Read the model definition and answer for the solid it produces. Units are mm, in the model's axes. A direction names the side the tool comes from. Coordinates: 2 decimals unless noted, no trailing zeros. Write each loop counter-clockwise with the first axis right and the second up, starting at its lowest first coordinate (ties: lowest second). Pieces come first, ordered by that corner, then holes. Notation, with made-up numbers: (-9, -15) -> (13, -15) arc R11 ccw to (13, 3) -> close; hole circle Ø6 at (-37.75, 82). An arc over 180 degrees is marked (long way). Write item = value, one per line. Start each with the question number.
1) For a pull along Y with two mould halves and no side action, classify faces 1 (the face through (0, 0, 0)), 2 (the face through (5, 14.5, -2)) as released by +Y, released by -Y, zero draft, split by the parting line, or undercut.
2) Find the intervals of material crossed by line 1 along Y through (x, z) = (-7, -5.25); line 2 along Z through (x, y) = (6.25, 7.75); line 3 along X through (y, z) = (5.25, 0.5), in increasing order. Write a range as from..to.
3) Section B-B (y = 20.25) is taken. Determine the outline of the cut face in (x, z).
4) Section A-A (y = 11.5) is taken. Determine the outline of the cut face in (x, z), plus the area to 3 significant figures.
5) Flat-ended cylindrical pins translate along their axes: pin 1 Ø3 at (y, z) = (4.5, -1) entering from +X; pin 2 Ø1.5 at (x, y) = (1, 14) entering from +Z; pin 3 Ø8 at (y, z) = (7, -7) entering from -X. Find the tip coordinate at first contact, or state that the pin passes through.
6) A tool of negligible diameter and unlimited length cuts with its end or side. For faces 3 (the face through (7.606, 21.05, 9.92)), 4 (the face through (-6.324, 16.965, -4.032)), 5 (the face through (3.83, 1.275, -9.237)), from which of +Z, -Z, +X, -X, +Y, -Y can it reach the whole face along a straight path? Write none if from no direction.
from build123d import *

# Parameters (mm, degrees)
DOME1_FACE_RADIUS = 12.5
DOME1_HEIGHT      = 1
FILLET1_R         = 1


with BuildPart() as part:
    # Sketch1 → Revolve1 (revolve)
    with BuildSketch(Plane.XY, mode=Mode.PRIVATE) as revolve1_sk:
        Polygon((0, 23.5), (12.5, 23.5), (12.5, 19.5), (7.5, 19.5), (7.5, 14.5), (5, 14.5), (5, 10), (8, 10), (8, 5), (10, 3), (10, 0), (0, 0), align=None)
    revolve(revolve1_sk.sketch.rotate(Axis((0, 0, 0), (0, 1, 0)), 90), axis=Axis((0, 0, 0), (0, 1, 0)))

    # Dome1: a dome of height H over a round flat face of radius A is a cap of a sphere of radius (A * A + H * H) / (2 * H)
    dome1_r = (DOME1_FACE_RADIUS * DOME1_FACE_RADIUS + DOME1_HEIGHT * DOME1_HEIGHT) / (2 * DOME1_HEIGHT)
    dome1_base = Plane((0, 23.5, 0), z_dir=(0, 1, 0))
    with Locations(dome1_base.offset(DOME1_HEIGHT - dome1_r)):
        dome1_ball = Sphere(dome1_r, mode=Mode.PRIVATE)
    add(split(dome1_ball, bisect_by=dome1_base, keep=Keep.TOP, mode=Mode.PRIVATE))

    # Fillet1
    fillet1_edges = [part.edges().sort_by_distance(p)[0] for p in [
        (12.5, 23.5, 0),
        (0, 3, 10),
        (0, 5, 8),
    ]]
    fillet(fillet1_edges, radius=FILLET1_R)


solid = part.part
Answer key:
q1.face_1 = released by -Y
q1.face_2 = undercut
q2.line_1 = 0..4.25, 19.5..24.01
q2.line_2 = -4.99..4.99
q2.line_3 = -8..8
q3.outline = circle Ø25 at (0, 0)
q4.outline = circle Ø10 at (0, 0)
q4.area = 78.5 mm^2
q5.pin_1 = 9.87
q5.pin_2 = 7.49
q5.pin_3 = -8.04
q6.face_3 = +Y, -Y
q6.face_4 = none
q6.face_5 = -Y
